Design review of the part built by this model. Coordinates are the model's own, in mm. Face numbers are marked on the shaded views. A direction names the side the tool comes from. Give positions to 0.01 mm unless a question says otherwise; leave off trailing zeros. Loops run counter-clockwise (first coordinate to the right, second up) from the corner with the lowest first, then second, coordinate; pieces in that order, holes last. Notation, with made-up numbers: (4.25, 23) -> (11.25, 23) arc R10 cw to (11.25, 41) -> close; hole circle Ø4 at (73, 15). An arc over 180 degrees is marked (long way). Answer in a Markdown table with one row per item. Add a question column.
(1) Consider section A-A on y = 0. Write out the cut boundary in (x, z), then the cut area to 3 significant figures.
(2) For the marked faces 1, 2, 3 and 4, list the 3-axis set-ups (+Z, -Z, +X, -X, +Y, -Y) from which the entire face can be reached by the end or side of a thin tool; tool diameter is ignored.
(3) Consider section C-C on y = 16. Write out the cut boundary in (x, z), then the cut area to 3 significant figures.
(4) For pin 1 (8 mm diameter, centred on x = 6, y = 19, fed in from -Z); pin 2 (15.5 mm diameter, centred on y = 0, z = 0, fed in from +X); pin 3 (2 mm diameter, centred on x = 4, z = 9, fed in from -Y); pin 4 (14.5 mm diameter, centred on y = -11.5, z = -4, fed in from +X), all flat-tipped, find the tip position at first contact; note any pin that passes through.
(5) Draft analysis for pull direction X (two halves, no side actions). For the marked faces 5, 6, 7 and 8, state which applies: +X half, -X half, draft (parallel to the pull), parting line (faces both ways), or undercut.
(6) For line 1 (X direction, y = -20, z = 10); line 2 (Y direction, x = -8.5, z = 0); line 3 (X direction, y = 8, z = -10), list the stretches that pass through material, from the lowest coordinate up.
(7) Consider section D-D on x = -6.25. Write out the cut boundary in (y, z).
(8) Consider section B-B on z = 0. Count the separate pieces of the cut face and the enclosed holes in it, then the cut area to 3 significant figures.
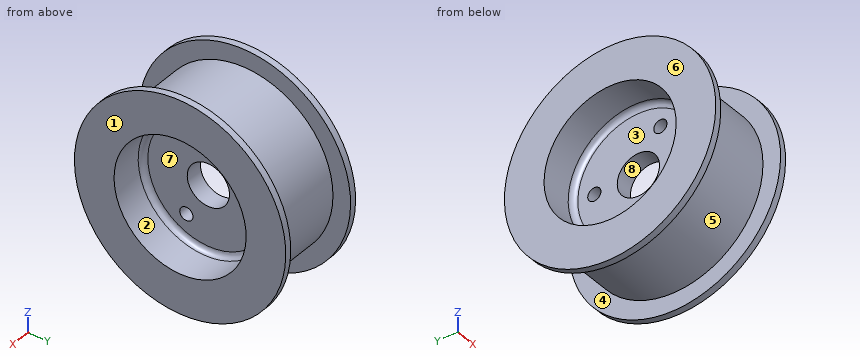
from build123d import *

# Parameters (mm, degrees)
SKETCH1_R           = 15
SKETCH1_R_2         = 4.8
SKETCH1_R_3         = 1.5
BOSS_EXTRUDE1_DEPTH = 2
SKETCH7_W           = 1.5
SKETCH7_H           = 4
FILLET1_R           = 1.25


with BuildPart() as part:
    # Sketch1 → Boss-Extrude1 (new, symmetric)
    with BuildSketch(Plane.YZ):
        with Locations(Location((0, 0, 0), (0, 0, 270))):
            Circle(SKETCH1_R)
        with Locations(Location((0, 0, 0), (0, 0, 270))):
            Circle(SKETCH1_R_2, mode=Mode.SUBTRACT)
        with Locations(Location((10, 0, 0), (0, 0, 270))):
            Circle(SKETCH1_R_3, mode=Mode.SUBTRACT)
        with Locations(Location((-5, -8.660254038, 0), (0, 0, 270))):
            Circle(SKETCH1_R_3, mode=Mode.SUBTRACT)
        with Locations(Location((-5, 8.660254038, 0), (0, 0, 270))):
            Circle(SKETCH1_R_3, mode=Mode.SUBTRACT)
    extrude(amount=BOSS_EXTRUDE1_DEPTH, both=True)

    # Sketch2 → Revolve1 (revolve)
    with BuildSketch(Plane(origin=(0, 0, 0), x_dir=(-1, 0, 0), z_dir=(0, 1, 0)), mode=Mode.PRIVATE) as revolve1_sk:
        Polygon((-2, 15), (-10.5, 15), (-10.5, 20), (10.5, 20), (10.5, 15), (2, 15), align=None)
    revolve(revolve1_sk.sketch.rotate(Axis((2, 0, 0), (-1, 0, 0)), 180), axis=Axis((2, 0, 0), (-1, 0, 0)))

    # Sketch7 → Revolve2 (revolve)
    with BuildSketch(Plane(origin=(0, 0, 0), x_dir=(-1, 0, 0), z_dir=(0, 1, 0)), mode=Mode.PRIVATE) as revolve2_sk:
        with Locations((-9.75, 22)):
            Rectangle(SKETCH7_W, SKETCH7_H)
    revolve2 = revolve(revolve2_sk.sketch.rotate(Axis((2, 0, 0), (-1, 0, 0)), 180), axis=Axis((2, 0, 0), (-1, 0, 0)))

    # Mirror1: Revolve2 across plane
    add(revolve2.mirror(Plane(origin=(0, 0, 0), x_dir=(0, 0, 1), z_dir=(1, 0, 0))))

    # Fillet1
    fillet1_edges = [part.edges().sort_by_distance(p)[0] for p in [
        (-2, 0, 15),
        (2, 0, 15),
    ]]
    fillet(fillet1_edges, radius=FILLET1_R)


solid = part.part
Values follow:
| question | item | result |
|---|---|---|
| 1 | outline | (-10.5, -24) -> (-9, -24) -> (-9, -20) -> (9, -20) -> (9, -24) -> (10.5, -24) -> (10.5, -15) -> (3.25, -15) arc R1.25 cw to (2, -13.75) -> (2, -4.8) -> (-2, -4.8) -> (-2, -13.75) arc R1.25 cw to (-3.25, -15) -> (-10.5, -15) -> close; (-10.5, 15) -> (-3.25, 15) arc R1.25 cw to (-2, 13.75) -> (-2, 4.8) -> (2, 4.8) -> (2, 13.75) arc R1.25 cw to (3.25, 15) -> (10.5, 15) -> (10.5, 24) -> (9, 24) -> (9, 20) -> (-9, 20) -> (-9, 24) -> (-10.5, 24) -> close |
| 1 | area | 317 mm2 |
| 2 | face 1 | +Z, -Z, +X, +Y, -Y |
| 2 | face 2 | +X |
| 2 | face 3 | -X |
| 2 | face 4 | none |
| 3 | outline | (-10.5, -17.89) -> (-9, -17.89) -> (-9, -12) -> (9, -12) -> (9, -17.89) -> (10.5, -17.89) -> (10.5, 17.89) -> (9, 17.89) -> (9, 12) -> (-9, 12) -> (-9, 17.89) -> (-10.5, 17.89) -> close |
| 3 | area | 539 mm2 |
| 4 | pin 1 | z = -17.57 |
| 4 | pin 2 | x = 2 |
| 4 | pin 3 | y = -18.33 |
| 4 | pin 4 | x = 10.5 |
| 5 | face 5 | undercut |
| 5 | face 6 | -X half |
| 5 | face 7 | +X half |
| 5 | face 8 | draft |
| 6 | line 1 | -10.5 to -9, 9 to 10.5 |
| 6 | line 2 | -20 to -15, 15 to 20 |
| 6 | line 3 | -2 to 2 |
| 7 | outline | circle Ø40 at (0, 0); hole circle Ø30 at (0, 0) |
| 8 | separate pieces | 3 |
| 8 | enclosed holes | 0 |
| 8 | area | 305 mm2 |
